Design review of the part shown in the three views and the two pictorial views. Dimensions are in mm from the part's minimum x, y and z. Coordinates: 2 decimals unless noted, no trailing zeros. Loops run counter-clockwise (first coordinate to the right, second up) from the corner with the lowest first, then second, coordinate; pieces in that order, holes last. Notation, with made-up numbers: M 86,-4.75 L 137,-4.75 A32 ccw 137,28.25 Z; hole C -7.5,-22 d4. An arc over 180 degrees is marked long. Answer as a JSON object with one key per item and string values. Group by question number.
Item 1: Add section B-B (y = 15.5). State the section outline as (x, z) points (1 decimal).
Item 2: Add section A-A (z = 1.7). State the section outline as (x, y) points (1 decimal), then the cut area to 3 significant figures.
Item 3: Add section C-C (x = 23). State the section outline as (y, z) points.
Item 4: Wall thickness on L1, parallel to X at y = 42.5, z = 4.3; L2, parallel to X at y = 13.5, z = 3.95 (1 decimal); L3, parallel to X at y = 30, z = 1.9 (1 decimal): over which ranges is each line inside the solid? List them lowest first. Write a range as from..to.
Item 5: Insertion check: pin 1 (1.5 mm diameter, centred on x = 75, z = 0.5, fed in from -Y); pin 2 (2 mm diameter, centred on x = 31.5, z = 0.5, fed in from -Y). Each pin has a flat end and moves straight along its axis. Give the tip position at first contact, or say it passes through.
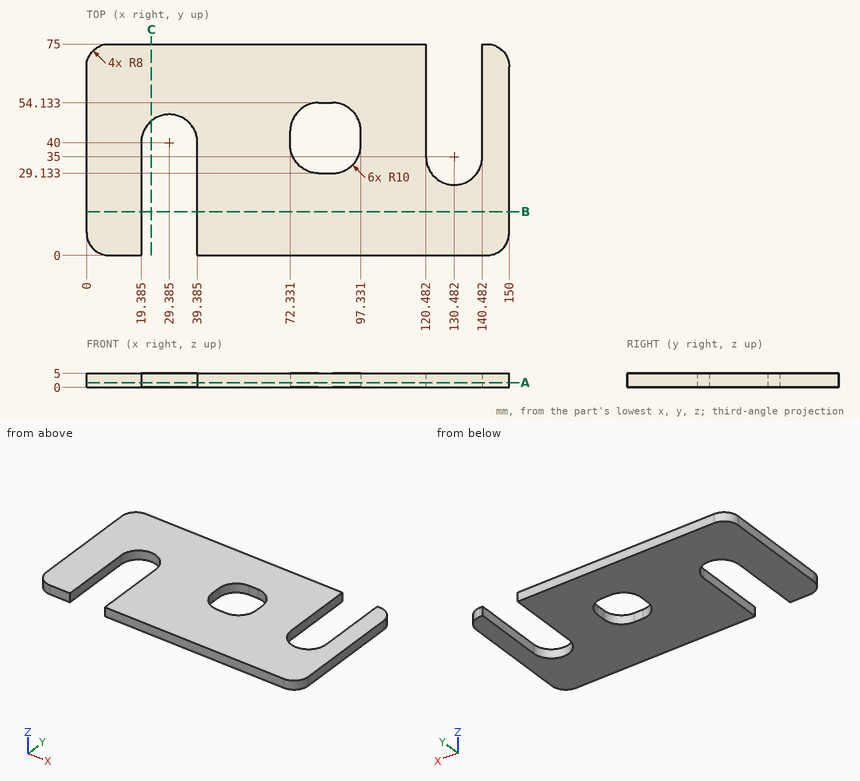
From the geometry:
{
 "1": {"outline": "M 0,0 L 19.4,0 L 19.4,5 L 0,5 Z; M 39.4,0 L 150,0 L 150,5 L 39.4,5 Z"},
 "2": {"outline": "M 0,8 A8 ccw 8,0 L 19.4,0 L 19.4,40 A10 cw 39.4,40 L 39.4,0 L 142,0 A8 ccw 150,8 L 150,67 A8 ccw 142,75 L 140.5,75 L 140.5,35 A10 cw 120.5,35 L 120.5,75 L 8,75 A8 ccw 0,67 Z; hole M 72.3,39.1 A10 ccw 82.3,29.1 L 87.3,29.1 A10 ccw 97.3,39.1 L 97.3,44.1 A10 ccw 87.3,54.1 L 82.3,54.1 A10 ccw 72.3,44.1 Z", "area": "8,740 mm²"},
 "3": {"outline": "M 47.7,0 L 75,0 L 75,5 L 47.7,5 Z"},
 "4": {"L1": "x = 0..19.7, 39.07..72.33, 97.33..120.48, 140.48..150", "L2": "x = 0..19.4, 39.4..150", "L3": "x = 0..19.4, 39.4..78.3, 91.4..121.8, 139.1..150"},
 "5": {"pin 1": "stops at y = 0", "pin 2": "stops at y = 49.5"}
}
